Here's how the part is built. I have some questions about the finished solid (model axes, mm). Face numbers are marked on the shaded views. A direction names the side the tool comes from. Round coordinates to 2 decimals unless told otherwise and drop trailing zeros. Loops run counter-clockwise (first coordinate to the right, second up) from the corner with the lowest first, then second, coordinate; pieces in that order, holes last. Notation, with made-up numbers: (-25, 67.25) - (25, 67.25) arc R28 ccw to (25, 93.25) - close; hole circle Ø2 at (25.5, -31.5). An arc over 180 degrees is marked (long way). Return JSON: item names as keys, results as strings. Group by question number.
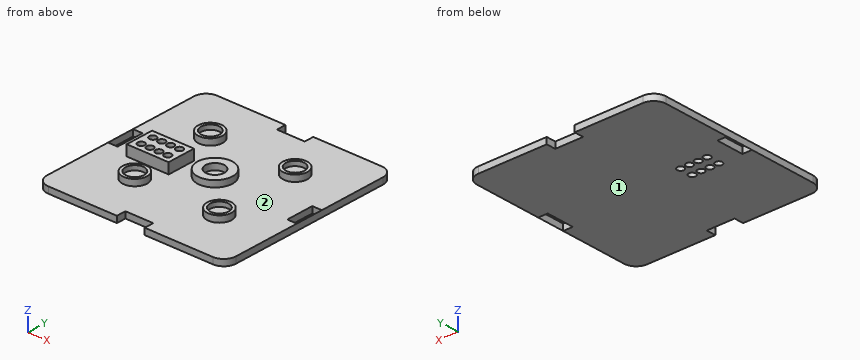
Autodesk Inventor part; units mm, degrees
sketch "Skizze1" plane through (27.583261, -56.113234, -10.899999) normal (0, 0, 1) x (1, 0, 0)
  line L0 (20.486741, 28.426785) -> (20.486741, 31.173234)
  line L1 (28.486738, 28.426785) -> (20.486741, 28.426785)
  line L2 (28.486738, 31.173234) -> (28.486738, 28.426785)
  circle A0 centre (48.116381, 27.672954) radius 3.500451
  line L3 (48.870292, 0.100002) -> (48.870292, 7.94323)
  line L4 (48.973479, 8.043232) -> (51.613555, 8.043232)
  line L5 (51.613555, 0) -> (48.973479, 0)
  circle A1 centre (48.116472, -19.586583) radius 3.50032
  line L6 (20.529933, -20.340319) -> (28.529944, -20.340319)
  line L7 (28.529944, -20.340319) -> (28.529944, -23.086762)
  line L8 (20.529933, -23.086762) -> (20.529933, -20.340319)
  circle A2 centre (0.857019, -19.586408) radius 3.500451
  line L9 (0.103188, 7.94323) -> (0.103188, 0.100002)
  line L10 (-2.640073, 8.043232) -> (0, 8.043232)
  line L11 (0, 0) -> (-2.640073, 0)
  circle A3 centre (0.856903, 27.67302) radius 3.50027
  circle A4 centre (6.691673, 3.973123) radius 1.000129
  circle A5 centre (9.236925, 3.973204) radius 1.000185
  circle A6 centre (11.781701, 3.973221) radius 0.999961
  circle A7 centre (14.326498, 3.973153) radius 0.999748
  circle A8 centre (14.3269, 0.233503) radius 0.99969
  circle A9 centre (11.78165, 0.233145) radius 1.000125
  circle A10 centre (9.236749, 0.233322) radius 0.999912
  circle A11 centre (6.691637, 0.232928) radius 1.000319
  line L12 (-2.640073, 8.043232) -> (0.103188, 8.043232)
  line L13 (0.103188, 8.043232) -> (0.103188, 0)
  line L14 (0.103188, 0) -> (-2.640073, 0)
  line L15 (20.486741, 31.173234) -> (20.486741, 28.426785)
  line L16 (28.486738, 28.426785) -> (28.486738, 31.173234)
  line L17 (48.116736, 31.173234) -> (28.486738, 31.173234)
  line L18 (0.85674, -23.086762) -> (20.529933, -23.086762)
  line L19 (-2.643261, 0.100002) -> (-2.643261, -19.586763)
  line L20 (51.616735, -19.586763) -> (51.616735, 0.100002)
  line L21 (-2.643261, 27.673233) -> (-2.643261, 7.94323)
  line L22 (20.486741, 31.173234) -> (0.85674, 31.173234)
  line L23 (51.616735, 7.94323) -> (51.616735, 27.673233)
  line L24 (28.529944, -23.086762) -> (48.116736, -23.086762)
  line L25 (-2.643261, -23.086762) -> (51.616735, -23.086762)
  line L26 (51.616735, -23.086762) -> (51.616735, 31.173234)
  line L27 (51.616735, 31.173234) -> (-2.643261, 31.173234)
  line L28 (-2.643261, 31.173234) -> (-2.643261, -23.086762)
  line L29 (51.613555, 8.043232) -> (48.870292, 8.043232)
  line L30 (48.870292, 8.043232) -> (48.870292, 0)
  line L31 (48.870292, 0) -> (51.613555, 0)
  line L32 (48.870292, 0) -> (51.613555, 0)
  line L33 (48.870292, 0) -> (48.870292, 8.043232)
  line L34 (51.613555, 8.043232) -> (48.870292, 8.043232)
  line L35 (48.870292, 8.043232) -> (48.870292, 0)
  line L36 (48.870292, 0) -> (51.613555, 0)
  line L37 (51.613555, 0) -> (51.613555, 8.043232)
  line L38 (0.103188, 0) -> (-2.640073, 0)
  line L39 (-2.640073, 8.043232) -> (0.103188, 8.043232)
  line L40 (0.103188, 0) -> (-2.640073, 0)
  line L41 (-2.640073, 0) -> (-2.640073, 8.043232)
  line L42 (-2.640073, 8.043232) -> (0.103188, 8.043232)
  line L43 (0.103188, 8.043232) -> (0.103188, 0)
  point P0 (-27.583261, 56.113234)
  point P1 (0.837182, 31.173234)
  point P2 (-2.643261, 27.700217)
  point P3 (-2.643261, -19.621008)
  point P4 (0.830931, -23.086762)
  point P5 (48.147826, -23.086762)
  point P6 (51.616735, -19.606381)
  point P7 (51.616735, 27.699042)
  point P8 (48.150981, 31.173234)
sketch "Skizze1 outline for Extrusion2" plane through (27.583261, -56.113234, -10.899999) normal (0, 0, 1) x (1, 0, 0)
  line L0 (28.486738, 28.426785) -> (20.486741, 28.426785)
  line L1 (28.486738, 31.173234) -> (28.486738, 28.426785)
  line L2 (20.486741, 28.426785) -> (20.486741, 31.173234)
  line L3 (48.116736, 31.173234) -> (28.486738, 31.173234)
  line L4 (20.486741, 31.173234) -> (0.85674, 31.173234)
  line L5 (48.150981, 31.173234) -> (48.116736, 31.173234)
  line L6 (0.85674, 31.173234) -> (0.837182, 31.173234)
  arc A0 (51.616735, 27.699042) -> (48.150981, 31.173234) centre (48.116381, 27.672954) ccw
  arc A1 (0.837182, 31.173234) -> (-2.643261, 27.700217) centre (0.856903, 27.67302) ccw
  line L7 (51.616735, 27.673233) -> (51.616735, 27.699042)
  line L8 (-2.643261, 27.700217) -> (-2.643261, 27.673233)
  line L9 (51.616735, 7.94323) -> (51.616735, 27.673233)
  line L10 (-2.643261, 27.673233) -> (-2.643261, 7.94323)
  line L11 (51.616735, 0.100002) -> (51.616735, 7.94323)
  line L12 (-2.643261, 7.94323) -> (-2.643261, 0.100002)
  line L13 (51.616735, -19.586763) -> (51.616735, 0.100002)
  line L14 (-2.643261, 0.100002) -> (-2.643261, -19.586763)
  line L15 (51.616735, -19.606381) -> (51.616735, -19.586763)
  line L16 (-2.643261, -19.586763) -> (-2.643261, -19.621008)
  arc A2 (48.147826, -23.086762) -> (51.616735, -19.606381) centre (48.116472, -19.586583) ccw
  arc A3 (-2.643261, -19.621008) -> (0.830931, -23.086762) centre (0.857019, -19.586408) ccw
  line L17 (48.116736, -23.086762) -> (48.147826, -23.086762)
  line L18 (0.830931, -23.086762) -> (0.85674, -23.086762)
  line L19 (28.529944, -23.086762) -> (48.116736, -23.086762)
  line L20 (0.85674, -23.086762) -> (20.529933, -23.086762)
  line L21 (28.529944, -20.340319) -> (28.529944, -23.086762)
  line L22 (20.529933, -23.086762) -> (20.529933, -20.340319)
  line L23 (20.529933, -20.340319) -> (28.529944, -20.340319)
  circle A4 centre (6.691637, 0.232928) radius 1.000319
  circle A5 centre (9.236749, 0.233322) radius 0.999912
  circle A6 centre (11.78165, 0.233145) radius 1.000125
  circle A7 centre (14.3269, 0.233503) radius 0.99969
  line L24 (-2.640073, 0) -> (-2.640073, 8.043232)
  line L25 (0, 0) -> (-2.640073, 0)
  line L26 (0.103188, 0) -> (0, 0)
  line L27 (0.103188, 0.100002) -> (0.103188, 0)
  line L28 (0.103188, 7.94323) -> (0.103188, 0.100002)
  line L29 (0.103188, 8.043232) -> (0.103188, 7.94323)
  line L30 (0, 8.043232) -> (0.103188, 8.043232)
  line L31 (-2.640073, 8.043232) -> (0, 8.043232)
  circle A8 centre (6.691673, 3.973123) radius 1.000129
  circle A9 centre (9.236925, 3.973204) radius 1.000185
  circle A10 centre (11.781701, 3.973221) radius 0.999961
  circle A11 centre (14.326498, 3.973153) radius 0.999748
  line L32 (51.613555, 8.043232) -> (51.613555, 0)
  line L33 (48.973479, 8.043232) -> (51.613555, 8.043232)
  line L34 (48.870292, 8.043232) -> (48.973479, 8.043232)
  line L35 (48.870292, 7.94323) -> (48.870292, 8.043232)
  line L36 (48.870292, 0.100002) -> (48.870292, 7.94323)
  line L37 (48.870292, 0) -> (48.870292, 0.100002)
  line L38 (48.973479, 0) -> (48.870292, 0)
  line L39 (51.613555, 0) -> (48.973479, 0)
extrude "Extrusion2" add sketch "Skizze1 outline for Extrusion2" along normal blind 1.8
sketch "Skizze2" plane through (27.583261, -56.113234, -9.099999) normal (0, 0, 1) x (1, 0, 0)
  line L0 (4.491739, -1.966767) -> (16.526742, -1.966767)
  line L1 (4.491739, -1.966767) -> (4.491739, 6.173234)
  line L2 (16.526742, 6.173234) -> (16.526742, -1.966767)
  line L3 (4.491739, 6.173234) -> (16.526742, 6.173234)
  line L4 (16.526742, -1.966767) -> (4.491739, -1.966767)
  circle A0 centre (9.236925, 3.973204) radius 1.000185
  circle A1 centre (11.781802, 3.973293) radius 1.000086
  circle A2 centre (14.32665, 3.9735) radius 1.00028
  circle A3 centre (14.326722, 0.233403) radius 0.999832
  circle A4 centre (11.78165, 0.233145) radius 1.000125
  circle A5 centre (9.236749, 0.233322) radius 0.999912
  circle A6 centre (6.691673, 3.973123) radius 1.000129
  circle A7 centre (6.691637, 0.232928) radius 1.000319
  point P0 (-27.583261, 56.113234)
extrude "Extrusion3" add sketch "Skizze2" along normal blind 3
sketch "Skizze3" plane through (27.583261, -56.113234, -9.099999) normal (0, 0, 1) x (1, 0, 0)
  circle A0 centre (12.321135, -8.122127) radius 2.666057
  circle A1 centre (12.321681, -8.121848) radius 3.499995
  circle A2 centre (12.3219, -8.121781) radius 2.666437
  circle A3 centre (12.321203, -8.121912) radius 3.500477
  circle A4 centre (24.486223, 4.041641) radius 4.998329
  circle A5 centre (24.486657, 4.043031) radius 2.66645
  circle A6 centre (36.651848, 16.208558) radius 2.666928
  circle A7 centre (36.651807, 16.208589) radius 3.500291
  line L0 (51.613555, 8.043232) -> (51.613555, 0)
  line L1 (51.613555, 4.021616) -> (-2.640073, 4.021616) construction
  line L2 (-2.640073, 0) -> (-2.640073, 8.043232)
  circle A8 centre (12.321135, 16.165359) radius 2.666057
  circle A9 centre (12.321203, 16.165144) radius 3.500477
  circle A10 centre (36.651848, -8.165326) radius 2.666928
  circle A11 centre (36.651807, -8.165357) radius 3.500291
  point P0 (-27.583261, 56.113234)
  point P1 (10.243668, -6.451202)
  point P2 (12.201311, -10.78549)
extrude "Extrusion4" add sketch "Skizze3" along normal blind 1.8
sketch "Skizze4" plane through (27.583261, -56.113234, -9.099999) normal (0, 0, 1) x (1, 0, 0)
  line L0 (51.616735, -19.606381) -> (51.616735, 27.699042) construction
  line L1 (51.616735, 4.04633) -> (-2.640073, 4.021616) construction
  line L2 (-2.640073, 0) -> (-2.640073, 8.043232) construction
  circle A0 centre (36.651848, 16.208558) radius 2.666928 construction
  circle A1 centre (36.651807, 16.208589) radius 3.500291 construction
  circle A2 centre (12.321681, -8.121848) radius 3.499995 construction
  arc A3 (12.201311, -10.78549) -> (10.243668, -6.451202) centre (12.3219, -8.121781) ccw construction
  arc A4 (10.243668, -6.451202) -> (12.201311, -10.78549) centre (12.321135, -8.122127) ccw construction
  circle A5 centre (24.486657, 4.043031) radius 2.66645 construction
  circle A6 centre (36.651848, 16.208558) radius 2.666928 construction
  arc A7 (10.243668, -6.451202) -> (12.201311, -10.78549) centre (12.321135, -8.122127) ccw construction
  arc A8 (12.201311, -10.78549) -> (10.243668, -6.451202) centre (12.3219, -8.121781) ccw construction
  point P0 (-27.583261, 56.113234)
sketch "Skizze5" plane through (39.904396, -39.947875, -9.099999) normal (0, 0, 1) x (1, 0, 0)
  circle A0 centre (0, 0) radius 2.666057
  circle A1 centre (24.330713, 0.043199) radius 2.666928
  circle A2 centre (24.330713, -24.330685) radius 2.666928
  arc A3 (-2.077467, -22.616561) -> (-0.119824, -26.950849) centre (0, -24.287486) ccw
  arc A4 (-0.119824, -26.950849) -> (-2.077467, -22.616561) centre (0.000765, -24.28714) ccw
  point P0 (-39.904396, 39.947875)
extrude "Extrusion5" add sketch "Skizze5" along normal blind 0.5
properties part number "brick_bottom_standard_block-0.5_circle-0,4"
Q1. Imagine slicing it at D-D, the plane y = -59. List the corners of the cut face in (x, z) for me, and give its area (3 significant figures).
Q2. Imagine slicing it at B-B, the plane x = 63.5. List the corners of the cut face in (y, z) for me, and give its area (3 significant figures).
Q3. Imagine slicing it at C-C, the plane x = 50.5. List the corners of the cut face in (y, z) for me, and give its area (3 significant figures).
Q4. Please list where these lines run through material, in increasing order: line 1 (X direction, y = -38.5, z = -7.8); line 2 (X direction, y = -65, z = -7.6); line 3 (Y direction, x = 66, z = -8.1).
Q5. For the marked faces 1 and 2, which set-ups out of +Z, -Z, +X, -X, +Y, -Y let a thin tool reach every point of the face, with its end or its side?
Q6. Will these pins go through, and if not, where does the flat tip stop? pin 1 Ø0.5 at (x, z) = (26.5, -10) entering from +Y; pin 2 Ø1 at (y, z) = (-43.5, -9) entering from -X; pin 3 Ø2 at (y, z) = (-27, -10) entering from -X; pin 4 Ø3 at (x, y) = (39.9, -39.95) entering from +Z.
Q7. Imagine slicing it at A-A, the plane y = -65.5. List the corners of the cut face in (x, z) for me.
Output values:
{
 "1": {"outline": "(24.94, -10.9) - (79.2, -10.9) - (79.2, -9.1) - (24.94, -9.1) - close", "area": "97.7 mm^2"},
 "2": {"outline": "(-79.2, -10.9) - (-24.94, -10.9) - (-24.94, -9.1) - (-36.48, -9.1) - (-36.48, -7.3) - (-37.34, -7.3) - (-37.34, -8.6) - (-42.47, -8.6) - (-42.47, -7.3) - (-43.33, -7.3) - (-43.33, -9.1) - (-60.86, -9.1) - (-60.86, -7.3) - (-61.71, -7.3) - (-61.71, -8.6) - (-66.84, -8.6) - (-66.84, -7.3) - (-67.7, -7.3) - (-67.7, -9.1) - (-79.2, -9.1) - close", "area": "109 mm^2"},
 "3": {"outline": "(-76.45, -10.9) - (-27.69, -10.9) - (-27.69, -9.1) - (-47.33, -9.1) - (-47.33, -7.3) - (-49.91, -7.3) - (-49.91, -9.1) - (-54.23, -9.1) - (-54.23, -7.3) - (-56.82, -7.3) - (-56.82, -9.1) - (-76.45, -9.1) - close", "area": "97.1 mm^2"},
 "4": {"line 1": "x = 36.72 to 37.67, 42.14 to 43.09, 61.03 to 61.97, 66.5 to 67.44", "line 2": "x = 36.49 to 37.35, 42.46 to 43.32, 60.81 to 61.67, 66.8 to 67.66", "line 3": "y = -67.3 to -66.28, -62.28 to -61.26, -42.93 to -41.9, -37.91 to -36.88"},
 "5": {"face 1": "-Z, +X, -X, +Y, -Y", "face 2": "+Z"},
 "6": {"pin 1": "stops at y = -25.38", "pin 2": "stops at x = 24.94", "pin 3": "stops at x = 24.97", "pin 4": "stops at z = -8.6"},
 "7": {"outline": "(24.94, -10.9) - (79.2, -10.9) - (79.2, -9.1) - (67.52, -9.1) - (67.52, -7.3) - (66.61, -7.3) - (66.61, -8.6) - (61.86, -8.6) - (61.86, -7.3) - (60.95, -7.3) - (60.95, -9.1) - (43.17, -9.1) - (43.17, -7.3) - (42.25, -7.3) - (42.25, -8.6) - (37.56, -8.6) - (37.56, -7.3) - (36.64, -7.3) - (36.64, -9.1) - (24.94, -9.1) - close"}
}
